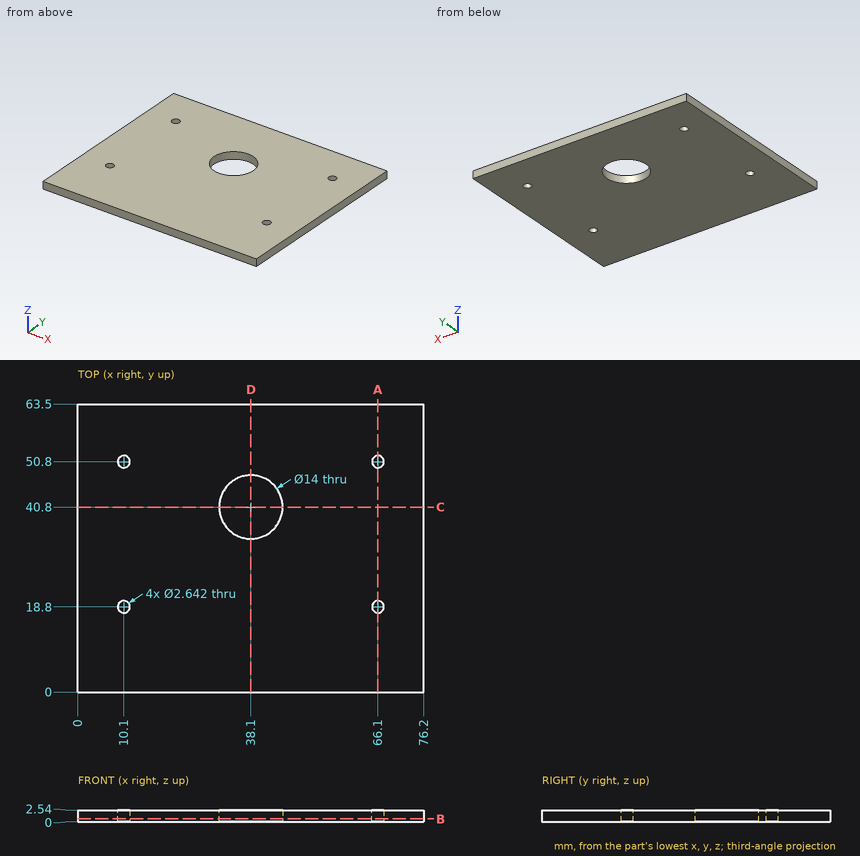
For this review, use the dimensioned drawing (mm, ordinates from the lowest corner) and the shaded views. Round coordinates to 2 decimals unless told otherwise and drop trailing zeros. Order: outer loops, then holes, each group sorted by start corner. A loop starts at its lowest first (then second) coordinate and runs counter-clockwise, first axis right, second up. Notation, with made-up numbers: (71, 47) -> (91, 47) arc R31 ccw to (91, 75) -> close; hole circle Ø8 at (-39.75, -13.5). An arc over 180 degrees is marked (long way). One line per item, written item: value. Start each with the question number.
Q1. Take a section at D-D (x = 38.1). Write out the cut boundary in (y, z), and give its area (3 significant figures).
Q2. Clearance check with a flat-ended pin moving along its axis: pin 1 Ø1.6 at (x, y) = (66.1, 50.8) entering from +Z. State where the tip first meets the part, or that it passes through.
Q3. Take a section at A-A (x = 66.1). Write out the cut boundary in (y, z), and give its area (3 significant figures).
Q4. Take a section at B-B (z = 0.6). Write out the cut boundary in (x, y).
Q5. Take a section at C-C (y = 40.8). Write out the cut boundary in (x, z), and give its area (3 significant figures).
Q6. Wall thickness on line 1 (Y direction, x = 10.1, z = 1.9); line 2 (X direction, y = 19, z = 1.65) (1 decimal); line 3 (Y direction, x = 38.1, z = 1.8): over which ranges is each line inside the solid? List them lowest first.
Reported:
1. outline: (0, 0) -> (33.8, 0) -> (33.8, 2.54) -> (0, 2.54) -> close; (47.8, 0) -> (63.5, 0) -> (63.5, 2.54) -> (47.8, 2.54) -> close
1. area: 126 mm2
2. pin 1: passes through
3. outline: (0, 0) -> (17.48, 0) -> (17.48, 2.54) -> (0, 2.54) -> close; (20.12, 0) -> (49.48, 0) -> (49.48, 2.54) -> (20.12, 2.54) -> close; (52.12, 0) -> (63.5, 0) -> (63.5, 2.54) -> (52.12, 2.54) -> close
3. area: 148 mm2
4. outline: (0, 0) -> (76.2, 0) -> (76.2, 63.5) -> (0, 63.5) -> close; hole circle Ø2.64 at (10.1, 18.8); hole circle Ø2.64 at (10.1, 50.8); hole circle Ø14 at (38.1, 40.8); hole circle Ø2.64 at (66.1, 18.8); hole circle Ø2.64 at (66.1, 50.8)
5. outline: (0, 0) -> (31.1, 0) -> (31.1, 2.54) -> (0, 2.54) -> close; (45.1, 0) -> (76.2, 0) -> (76.2, 2.54) -> (45.1, 2.54) -> close
5. area: 158 mm2
6. line 1: y = 0 to 17.48, 20.12 to 49.48, 52.12 to 63.5
6. line 2: x = 0 to 8.8, 11.4 to 64.8, 67.4 to 76.2
6. line 3: y = 0 to 33.8, 47.8 to 63.5
